Model file for the job. Use its own axes, mm. Face numbers are marked on the shaded views. A direction names the side the tool comes from. Round coordinates to 2 decimals unless told otherwise and drop trailing zeros. Order: outer loops, then holes, each group sorted by start corner. A loop starts at its lowest first (then second) coordinate and runs counter-clockwise, first axis right, second up. Notation, with made-up numbers: (65, 46) - (110, 46) arc R13 cw to (110, 63) - close; hole circle Ø2 at (19.5, -33). An arc over 180 degrees is marked (long way). Put each result on its own line as item: value. Start each with the question number.
Item 1: Saw through at C-C on x = -47. List the corners of the cut face in (y, z).
Item 2: Probe probe 1 along Y at (x, z) = (-66, -87); probe 2 along Y at (x, z) = (-239.5, 15.5); probe 3 along Z at (x, y) = (-181, 124). List the from-to ranges inside material, lowest first.
Item 3: Saw through at A-A on z = -113. List the corners of the cut face in (x, y).
Item 4: Pin check, flat tips, straight feed: pin 1 Ø12 at (x, z) = (-178.5, -51) entering from -Y; pin 2 Ø5 at (x, z) = (-220.5, -108) entering from -Y; pin 3 Ø1 at (x, z) = (-65, -111) entering from +Y; pin 4 Ø1.5 at (x, y) = (-152.5, 67) entering from -Z. Stop position of each tip, or through.
Item 5: Saw through at B-B on y = 25. List the corners of the cut face in (x, z), plus the area to 3 significant figures.
Item 6: Mould opens along Z. For the marked faces 3, 4 and 5 say: pulls with the +Z half, pulls with the -Z half, needs draft (parallel to the pull), parting line crosses it, or undercut.
Item 7: Saw through at D-D on z = -68.5. List the corners of the cut face in (x, y).
Item 8: Which spindle directions (+Z, -Z, +X, -X, +Y, -Y) get a long thin tool onto all of the face, cutting with end or side? Do the marked faces 1 and 2. Say none if no direction does.
```python
from build123d import *

# Parameters (mm, degrees)
F0_W       = 76.0625377297
F0_H       = 98.9513029344
F1_DEPTH   = 172.974
F2_R       = 16.4981826782
F3_DEPTH   = 207.518
F1_FACE_W  = 76.0625377297
F1_FACE_H  = 172.974
F1_FACE1_W = 76.0625377297
F1_FACE1_H = 172.974
F6_R       = 83.6259605226
F7_DEPTH   = 25.4


with BuildPart() as f1:
    # F0 (on Front) → F1 (new body)
    with BuildSketch(Plane.XZ):
        with Locations((-140.9135572612, -56.9459532853)):
            Rectangle(F0_W, F0_H)
    extrude(amount=-F1_DEPTH)

    # F2 (on Right) → F3 (cut)
    with BuildSketch(Plane.YZ):
        with Locations((32.9360701144, -37.6199260354)):
            Circle(F2_R)
    extrude(amount=-F3_DEPTH, mode=Mode.SUBTRACT)

    # F1_face (on face) → F4 (revolve)
    with BuildSketch(Plane(origin=(-140.9135572612, 86.487, -106.4216047525), x_dir=(1, 0, 0), z_dir=(0, 0, -1))):
        Rectangle(F1_FACE_W, F1_FACE_H)
    revolve(axis=Axis((-178.9448261261, 86.487, -106.4216047525), (0, -1, 0)))

    # F1_face1 (on face) → F5 (revolve)
    with BuildSketch(Plane(origin=(-140.9135572612, 86.487, -7.4703018181), x_dir=(1, 0, 0), z_dir=(0, 0, 1))):
        Rectangle(F1_FACE1_W, F1_FACE1_H)
    revolve(axis=Axis((-178.9448261261, 86.487, -7.4703018181), (0, -1, 0)))

    # F6 (on Front) → F7 (join)
    with BuildSketch(Plane.XZ):
        with Locations((-92.7199497819, -53.7736974657)):
            Circle(F6_R)
    extrude(amount=F7_DEPTH)


solid = f1.part
```
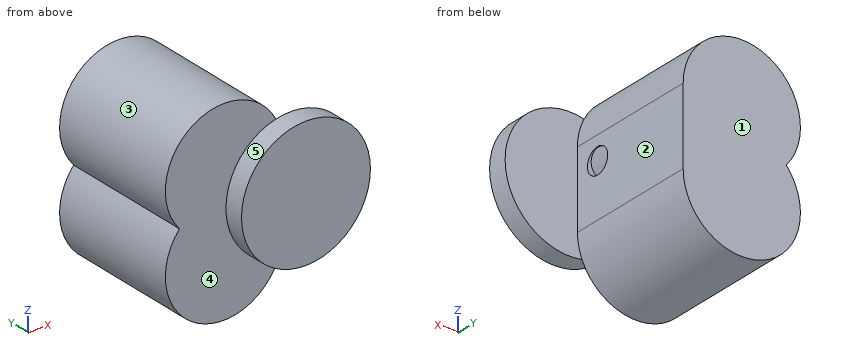
Results found:
1. outline: (-25.4, -123.8) - (0, -123.8) - (0, 16.25) - (-25.4, 16.25) - close
2. probe 1: y = -25.4 to 0
2. probe 2: y = 0 to 172.97
2. probe 3: z = -182.46 to 68.56
3. outline: (-254.72, 0) - (-151.76, 0) - (-151.76, -25.4) - (-33.68, -25.4) - (-33.68, 0) - (-103.17, 0) - (-103.17, 172.97) - (-254.72, 172.97) - close
4. pin 1: stops at y = -25.4
4. pin 2: stops at y = 0
4. pin 3: stops at y = 0
4. pin 4: stops at z = -178.01
5. outline: (-236.72, -56.95) arc R76.06 ccw (long way) to (-102.88, -106.42) - (-102.88, -52.08) - (-117.34, -52.08) arc R76.06 ccw to (-104.52, -23.16) - (-102.88, -23.16) - (-102.88, -7.47) arc R76.06 ccw (long way) to start
5. area: 32,500 mm²
6. face 3: undercut
6. face 4: needs draft
6. face 5: parting line crosses it
7. outline: (-244.88, 0) - (-175.04, 0) - (-175.04, -25.4) - (-10.4, -25.4) - (-10.4, 0) - (-102.88, 0) - (-102.88, 172.97) - (-244.88, 172.97) - close
8. face 1: +Z, -Z, +X, -X, +Y
8. face 2: +Z, -Z, +X, +Y
